```python
from build123d import *

# Parameters (mm, degrees)
SKETCH1_R           = 10.795
BOSS_EXTRUDE1_DEPTH = 3.175
SKETCH2_R           = 6.35
BOSS_EXTRUDE2_DEPTH = 12.7
SKETCH3_W           = 3.175
SKETCH3_H           = 25.4
CUT_EXTRUDE1_DEPTH  = 3.175


with BuildPart() as part:
    # Sketch1 → Boss-Extrude1 (new, symmetric)
    with BuildSketch(Plane.XY):
        Circle(SKETCH1_R)
    extrude(amount=BOSS_EXTRUDE1_DEPTH, both=True)

    # Sketch2 → Boss-Extrude2 (add)
    with BuildSketch(Plane(origin=(0, 0, -3.175), x_dir=(-1, 0, 0), z_dir=(0, 0, -1))):
        Circle(SKETCH2_R)
    extrude(amount=BOSS_EXTRUDE2_DEPTH)

    # Sketch3 → Cut-Extrude1 (cut)
    with BuildSketch(Plane.XY.offset(3.175)):
        Rectangle(SKETCH3_W, SKETCH3_H)
    extrude(amount=-CUT_EXTRUDE1_DEPTH, mode=Mode.SUBTRACT)


solid = part.part
```
Source: CAD feature listing. Evaluate the final solid. Frame: model axes, mm. A direction names the side the tool comes from. Give positions to 0.01 mm unless a question says otherwise; leave off trailing zeros. Loops run counter-clockwise (first coordinate to the right, second up) from the corner with the lowest first, then second, coordinate; pieces in that order, holes last. Notation, with made-up numbers: (12, 80.5) -> (64, 80.5) arc R29 ccw to (64, 118.5) -> close; hole circle Ø8 at (38, 36.25). An arc over 180 degrees is marked (long way). Put each result on its own line as item: value. Start each with the question number.
1) Reachability of faces 1 (the face through (0, 0, -15.875)), 2 (the face through (0, 0, 0)), 3 (the face through (5, -5, -3.175)) from +Z, -Z, +X, -X, +Y, -Y: full face, straight path, thin tool, end or side. Return the list, or none.
2) Cut plane B-B (x = 0). Return loops of the section in (y, z) (3 decimals).
3) Contact query for flat-ended pins moving along their axis: P1, Ø1, axis at y = 4.5, z = 2, coming from the -X side; P2, Ø1.5, axis at y = 6.5, z = -6, coming from the +X side; P3, Ø3, axis at y = -5.5, z = -8.5, coming from the -X side. Output: stop coordinate, or through.
4) Draft query along X for faces 4 (the face through (-2.34, -10.54, 0.04)), 5 (the face through (1.588, 0, 2)), 6 (the face through (-5, 0, 3.175)). Return one class per face: released by +X, released by -X, zero draft, split by the parting line, or undercut.
5) Material intervals for probe 1 along Z at (x, y) = (5.5, 5.5) (3 decimals); probe 2 along X at (y, z) = (5.25, -11); probe 3 along X at (y, z) = (-2.5, -7.25), sorted ascending.
6) Cut plane D-D (y = 3.75). Return loops of the section in (x, z) (1 decimal).
7) Cut plane C-C (z = -1). Return loops of the section in (x, y) (3 decimals), then the cut area to 3 significant figures.
Results are:
1. face 1: -Z, +X, -X, +Y, -Y
1. face 2: +Z, +Y, -Y
1. face 3: -Z
2. outline: (-10.795, -3.175) -> (-6.35, -3.175) -> (-6.35, -15.875) -> (6.35, -15.875) -> (6.35, -3.175) -> (10.795, -3.175) -> (10.795, 0) -> (-10.795, 0) -> close
3. P1: stops at x = -10.03
3. P2: stops at x = 2.69
3. P3: stops at x = -4.93
4. face 4: split by the parting line
4. face 5: undercut
4. face 6: zero draft
5. probe 1: z = -3.175 to 3.175
5. probe 2: x = -3.57 to 3.57
5. probe 3: x = -5.84 to 5.84
6. outline: (-10.1, -3.2) -> (-5.1, -3.2) -> (-5.1, -15.9) -> (5.1, -15.9) -> (5.1, -3.2) -> (10.1, -3.2) -> (10.1, 3.2) -> (1.6, 3.2) -> (1.6, 0) -> (-1.6, 0) -> (-1.6, 3.2) -> (-10.1, 3.2) -> close
7. outline: circle Ø21.59 at (0, 0)
7. area: 366 mm2
